Check sheet for the modelled part. Datum: model origin and axes. Units: mm. A direction names the side the tool comes from. Round coordinates to 2 decimals unless told otherwise and drop trailing zeros. Write each loop counter-clockwise with the first axis right and the second up, starting at its lowest first coordinate (ties: lowest second). Pieces come first, ordered by that corner, then holes. Notation, with made-up numbers: (19.25, -19.5) - (67.25, -19.5) arc R7 ccw to (67.25, -15.5) - close; hole circle Ø4 at (-33, 11.25). An arc over 180 degrees is marked (long way). Use one line per item in the form item = value. Start each with the question number.
1) Scan lines: probe 1 along Z at (x, y) = (13.75, 0); probe 2 along Z at (x, y) = (18.5, 0); probe 3 along Z at (x, y) = (16.5, 6.5). Record each from-to range of solid material in increasing order.
2) Draft check along Z on faces 3 (the face through (12.675, -1.432, 150.906)), 4 (the face through (19, -3.8, 7.3)). Enter one of: +Z half, -Z half, draft (parallel to the pull), parting line (faces both ways), or undercut.
3) Gauge pin test, flat ends, axial feed: P1, Ø3, axis at x = 14.5, y = 9.5, coming from the -Z side; P2, Ø2, axis at x = 17, z = 129, coming from the -Y side; P3, Ø4, axis at x = 12.5, y = -15.5, coming from the -Z side; P4, Ø13, axis at y = 0, z = 140, coming from the +X side. Record the tip position at first contact, or that the pin passes through.
4) Section check B-B (y = 0). Count the separate pieces of the cut face and the enclosed holes in it, then the cut area to 3 significant figures.
5) Set-up check for faces 1 (the face through (9.63, -1.73, -7.81)), 2 (the face through (9.37, -3.47, -15.62)): record each of +Z, -Z, +X, -X, +Y, -Y from which the full face is reachable in a straight line by a thin tool's end or side.
6) Section check A-A (z = 140). Record the boundary of the cut face in (x, y).
from build123d import *

# Parameters (mm, degrees)
F0_R      = 16
F0_R_2    = 8
F1_DEPTH  = 19
F0_R_3    = 24
F0_R_4    = 11
F2_DEPTH  = 25
F4_R      = 11
F5_DEPTH  = 25
F6_R      = 11
F10_DEPTH = 25.0010001
F11_R     = 8
F12_DEPTH = 19.0010001


with BuildPart() as f1:
    # F0 (on Right) → F1 (new body)
    with BuildSketch(Plane.YZ):
        Circle(F0_R)
        Circle(F0_R_2, mode=Mode.SUBTRACT)
        Circle(F0_R_2)
    extrude(amount=F1_DEPTH)



with BuildPart() as f2:
    # F0 (on Right) → F2 (new body)
    with BuildSketch(Plane.YZ):
        with Locations((0, 140)):
            Circle(F0_R_3)
        with Locations((0, 140)):
            Circle(F0_R_4, mode=Mode.SUBTRACT)
    extrude(amount=F2_DEPTH)


with BuildPart() as f5:
    # F4 (on face) → F5 (new body)
    with BuildSketch(Plane.YZ.offset(25)):
        with Locations((0, 140)):
            Circle(F4_R)
    extrude(amount=-F5_DEPTH)


with BuildPart() as f1_1:
    add(f1.part)

    add(f2.part)  # F9 merges F2

    add(f5.part)  # F9 merges F5
    # F8 (on plane+point) → F9 section 0
    with BuildSketch(Plane.XY.offset(140)):
        with BuildLine():
            add(Edge.make_bspline(
                [(9, -24), (19.3923048454, -24), (14.1961524227, 12), (9, 48), (3.8038475773, 12), (-1.3923048454, -24), (9, -24)],
                knots=[0, 0, 0, 2.0943951024, 2.0943951024, 4.1887902048, 4.1887902048, 6.2831853072, 6.2831853072, 6.2831853072], degree=2, weights=[1, 0.5, 1, 0.5, 1, 0.5, 1]))
        make_face()
    # F3 (on Top) → F9 section 1
    with BuildSketch(Plane.XY):
        with BuildLine():
            add(Edge.make_bspline(
                [(9, -16), (19.3923048454, -16), (14.1961524227, 8), (9, 32), (3.8038475773, 8), (-1.3923048454, -16), (9, -16)],
                knots=[0, 0, 0, 2.0943951024, 2.0943951024, 4.1887902048, 4.1887902048, 6.2831853072, 6.2831853072, 6.2831853072], degree=2, weights=[1, 0.5, 1, 0.5, 1, 0.5, 1]))
        make_face()
    loft()

    # F6 (on face) → F10 (cut, through all)
    with BuildSketch(Plane.YZ.offset(25)):
        with Locations((0, 140)):
            Circle(F6_R)
    extrude(amount=-F10_DEPTH, mode=Mode.SUBTRACT)

    # F11 (on face) → F12 (cut, through all)
    with BuildSketch(Plane.YZ.offset(19)):
        Circle(F11_R)
    extrude(amount=-F12_DEPTH, mode=Mode.SUBTRACT)


solid = f1_1.part
Results are:
q1.probe_1 = -16 to -8, 8 to 129, 151 to 164
q1.probe_2 = -16 to -8, 8 to 16, 116 to 129, 151 to 164
q1.probe_3 = -14.62 to -4.66, 4.66 to 14.62, 116.9 to 131.13, 148.87 to 163.1
q2.face_3 = undercut
q2.face_4 = draft
q3.P1 = -13.86
q3.P2 = -21.82
q3.P3 = -8.59
q3.P4 = through
q4.separate_pieces = 3
q4.enclosed_holes = 0
q4.area = 2,150 mm²
q5.face_1 = +X, -X
q5.face_2 = none
q6.outline = (0, -24) - (25, -24) - (25, -11) - (0, -11) - close; (0, 11) - (25, 11) - (25, 24) - (0, 24) - close
